Autodesk Inventor part; units mm, degrees
ref_plane "Work Plane1" through (0, 0, 101.6) normal (0, 0, 1) x (1, 0, 0)
ref_plane "YZ Plane" through (0, 0, 0) normal (1, 0, 0) x (0, 1, 0)
ref_plane "XZ Plane" through (0, 0, 0) normal (0, 1, 0) x (-1, 0, 0)
sketch "Sketch1" plane through (0, 0, 0) normal (0, 0, 1) x (1, 0, 0)
  line L0 (-2.4289, 0) -> (-2.4289, 12.7)
  line L1 (-2.4289, 12.7) -> (-4.0164, 12.7)
  line L2 (-4.0164, 12.7) -> (-4.0164, 0)
  line L3 (-4.0164, 0) -> (-29.4164, 0) construction
  line L4 (-33.2939, -14.2875) -> (-33.2939, -12.7)
  line L5 (-33.2939, -12.7) -> (-16.7164, -12.7)
  line L6 (-16.7164, -14.2875) -> (-33.2939, -14.2875)
  arc A0 (-16.7164, -14.2875) -> (-2.4289, 0) centre (-16.7164, 0) ccw
  arc A1 (-16.7164, -12.7) -> (-4.0164, 0) centre (-16.7164, 0) ccw
  dimension "d5" = 1.5875
  dimension "d9" = 1.5875
extrude "Extrusion1" add sketch "Sketch1" along normal blind 127
ref_plane "Work Plane1" through (0, 0, 101.6) normal (0, 0, 1) x (1, 0, 0)
sketch "Sketch2" plane through (0, 0, 101.6) normal (0, 0, 1) x (1, 0, 0)
  arc A0 (-16.7164, -14.2875) -> (-2.4289, 0) centre (-16.7164, 0) ccw
  arc A1 (-16.7164, -14.2875) -> (-2.4289, 0) centre (-16.7164, 0) ccw
  line L0 (-0.8414, 0) -> (-0.8414, 6.35)
  line L1 (-0.8414, 6.35) -> (-2.4289, 6.35)
  line L2 (-2.4289, 0) -> (-2.4289, 12.7)
  line L3 (-16.7164, -15.875) -> (-23.0664, -15.875)
  line L4 (-23.0664, -15.875) -> (-23.0664, -14.2875)
  line L5 (-16.7164, -14.2875) -> (-33.2939, -14.2875)
  line L6 (-23.0664, -14.2875) -> (-16.7164, -14.2875)
  line L7 (-2.4289, 6.35) -> (-2.4289, 0)
  arc A2 (-16.7164, -15.875) -> (-0.8414, 0) centre (-16.7164, 0) ccw
  line L8 (-16.7164, 0) -> (-16.7164, -14.2875) construction
  line L9 (-16.7164, -15.875) -> (-16.7164, -20.4579) construction
  point P0 (0, 0)
  dimension "d14" = 6.35
  dimension "d15" = 6.35
extrude "Extrusion2" add sketch "Sketch2" against normal blind 3.175
fillet "Fillet1" radius 1.5875 8 edges at (-0.8414, 6.35, 100.0125) (-5.4911, -11.2253, 101.6) (-0.8414, 3.175, 101.6) (-19.8914, -15.875, 101.6) (-5.4911, -11.2253, 98.425) (-0.8414, 3.175, 98.425) (-19.8914, -15.875, 98.425) (-23.0664, -15.875, 100.0125)
pattern_linear "Rectangular Pattern1" count 4 spacing 25.4 along (0, 0, -1) of "Extrusion2", "Fillet1"
properties part number "Grip"
Read the model definition and answer for the solid it produces. Units are mm, in the model's axes. A direction names the side the tool comes from. Round coordinates to 2 decimals unless told otherwise and drop trailing zeros. Write each loop counter-clockwise with the first axis right and the second up, starting at its lowest first coordinate (ties: lowest second). Pieces come first, ordered by that corner, then holes. Notation, with made-up numbers: M -25,-23.5 L -4,-23.5 A19 ccw -4,-12.5 Z; hole C -22,29 d6. An arc over 180 degrees is marked long. Use a Markdown table: item, result.
1) The part is cut by section B-B (z = 80). Write down the section's boundary in (x, y) (1 decimal).
Answers follow:
| item | result |
|---|---|
| outline | M -33.3,-14.3 L -16.7,-14.3 A14.3 ccw -2.4,0 L -2.4,12.7 L -4,12.7 L -4,0 A12.7 cw -16.7,-12.7 L -33.3,-12.7 Z |
2) Flat-ended cylindrical pins translate along their axes: pin 1 (8.5 mm diameter, centred on x = -28.5, z = 74.5, fed in from +Y); pin 2 (2 mm diameter, centred on y = -10, z = 106.5, fed in from +X); pin 3 (6 mm diameter, centred on x = -14, y = -9, fed in from +Z); pin 4 (2 mm diameter, centred on y = -1, z = 70, fed in from +X). Find the tip coordinate at first contact, or state that the pin passes through.
Answers follow:
| item | result |
|---|---|
| pin 1 | stops at y = -12.7 |
| pin 2 | stops at x = -5.62 |
| pin 3 | passes through |
| pin 4 | stops at x = -2.43 |
3) For a pull along Z with two mould halves and no side action, classify faces 1 (the flat face through (-25, -12.7, 63)), 2 (the flat face through (-2.429, 6, 63)) as pulls with the +Z half, pulls with the -Z half, needs draft (parallel to the pull), parting line crosses it, or undercut.
Answers follow:
| item | result |
|---|---|
| face 1 | needs draft |
| face 2 | undercut |
4) Straight lines are drawn through the part: line 1 along X through (y, z) = (7, 115); line 2 along Y through (x, z) = (-30.5, 79); line 3 along X through (y, z) = (-9.5, 108). For each, find the intervals that lie inside material, in ascending order. Write a range as [from, to].
Answers follow:
| item | result |
|---|---|
| line 1 | x = [-4.02, -2.43] |
| line 2 | y = [-14.29, -12.7] |
| line 3 | x = [-8.29, -6.04] |
5) A tool of negligible diameter and unlimited length cuts with its end or side. For faces 3 (the cylindrical face through (-7.638, -8.881, 62.611)), 4 (the cylindrical face through (-6.5, -9.99, 87.16)), 5 (the cylindrical face through (-6.5, -9.99, 10.96)), 6 (the cylindrical face through (-6.5, -9.99, 114.12)), from which of +Z, -Z, +X, -X, +Y, -Y can it reach the whole face along a straight path? Write none if from no direction.
Answers follow:
| item | result |
|---|---|
| face 3 | +Z, -Z, -X, +Y |
| face 4 | +X, -Y |
| face 5 | -Z, +X, -Y |
| face 6 | +Z, +X, -Y |
6) The part is cut by section C-C (x = -26). Write down the section's boundary in (y, z), plus the area to 3 significant figures.
Answers follow:
| item | result |
|---|---|
| outline | M -14.29,0 L -12.7,0 L -12.7,127 L -14.29,127 Z |
| area | 202 mm2 |
